Design review of the part shown in the three views and the two pictorial views. Dimensions are in mm from the part's minimum x, y and z. A direction names the side the tool comes from. Give positions to 0.01 mm unless a question says otherwise; leave off trailing zeros. Loops run counter-clockwise (first coordinate to the right, second up) from the corner with the lowest first, then second, coordinate; pieces in that order, holes last. Notation, with made-up numbers: (82, 35.25) -> (124, 35.25) arc R22 ccw to (124, 72.25) -> close; hole circle Ø4 at (81.5, -14). An arc over 180 degrees is marked (long way). Answer as CSV lines item,"result". Start each with the question number.
Item 1: For L1, parallel to X at y = 7.75, z = 19; L2, parallel to Z at x = 17.5, y = 28.75, list the stretches that pass through material, from the lowest coordinate up. Write a range as from..to.
Item 2: Machinability: for the marked faces 1 and 2, which of the approach directions +Z, -Z, +X, -X, +Y, -Y give a long, thin tool a straight path to every point of the face, cutting with its end or side? Answer none if there is none.
Item 3: Add section D-D on z = 8. State the section outline as (x, y) points, plus the area to 3 significant figures.
Item 4: The part is to be moulded in two halves that separate along X. For the marked faces 3, 4, 5 and 6, say which applies: +X half, -X half, draft (parallel to the pull), parting line (faces both ways), or undercut.
Item 5: Add section A-A on y = 18. State the section outline as (x, z) points, plus the area to 3 significant figures.
Item 6: Clearance check with flat-ended pins moving along their axes: P1, Ø5, axis at x = 27.5, z = 24.5, coming from the -Y side; P2, Ø20, axis at x = 14.5, z = 23, coming from the -Y side. State where each tip first meets the part, or that it passes through.
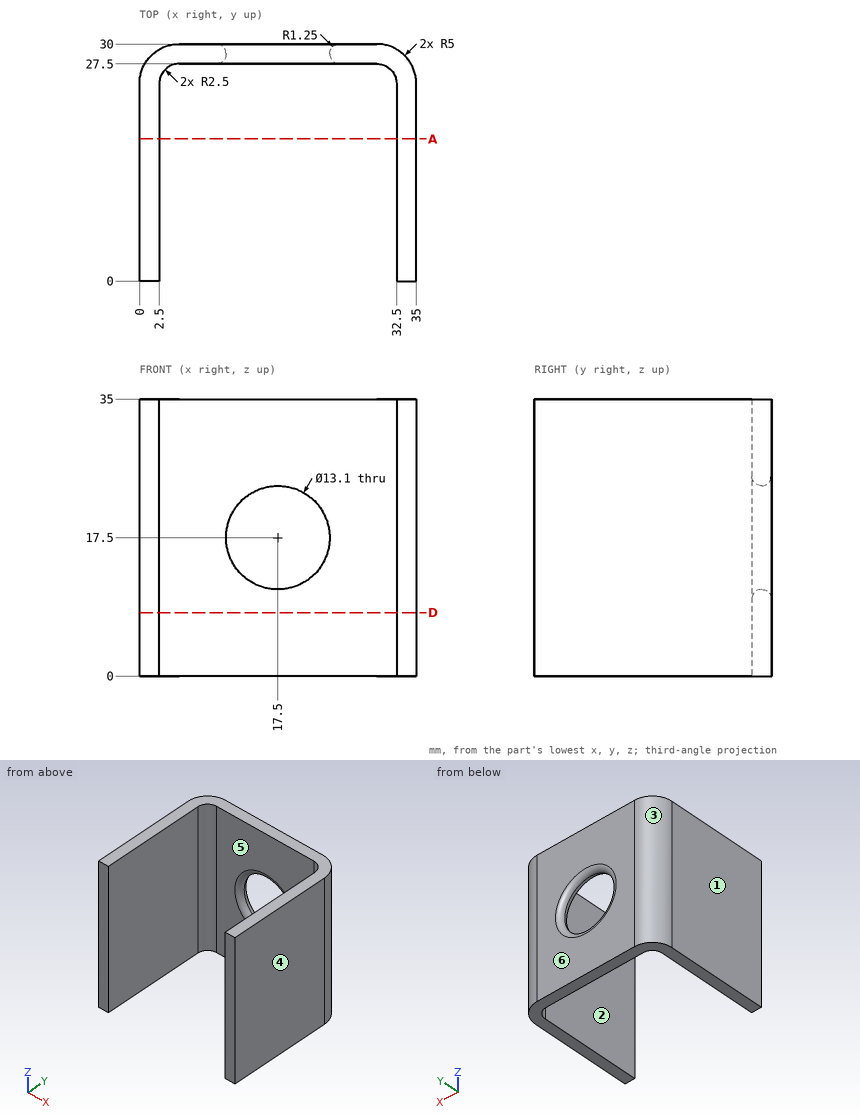
Computed values:
1,L1,"0..2.5, 32.5..35"
1,L2,"0..10.95, 24.05..35"
2,face 1,"+Z, -Z, -X, +Y, -Y"
2,face 2,"+Z, -Z, -Y"
3,outline,"(0, 0) -> (2.5, 0) -> (2.5, 25) arc R2.5 cw to (5, 27.5) -> (30, 27.5) arc R2.5 cw to (32.5, 25) -> (32.5, 0) -> (35, 0) -> (35, 25) arc R5 ccw to (30, 30) -> (5, 30) arc R5 ccw to (0, 25) -> close"
3,area,"217 mm²"
4,face 3,"-X half"
4,face 4,"+X half"
4,face 5,"undercut"
4,face 6,"draft"
5,outline,"(0, 0) -> (2.5, 0) -> (2.5, 35) -> (0, 35) -> close; (32.5, 0) -> (35, 0) -> (35, 35) -> (32.5, 35) -> close"
5,area,"175 mm²"
6,P1,"y = 27.5"
6,P2,"y = 27.45"
